Could you check a few things on this model? Use its own coordinates, in mm. Face numbers are marked on the shaded views. A direction names the side the tool comes from. Coordinates: 2 decimals unless noted, no trailing zeros. Order: outer loops, then holes, each group sorted by start corner. A loop starts at its lowest first (then second) coordinate and runs counter-clockwise, first axis right, second up. Notation, with made-up numbers: M 26,25.5 L 54,25.5 A32 ccw 54,52.5 Z; hole C -9,39 d3. An arc over 180 degrees is marked long. Write item = value, one per line. Start each with the question number.
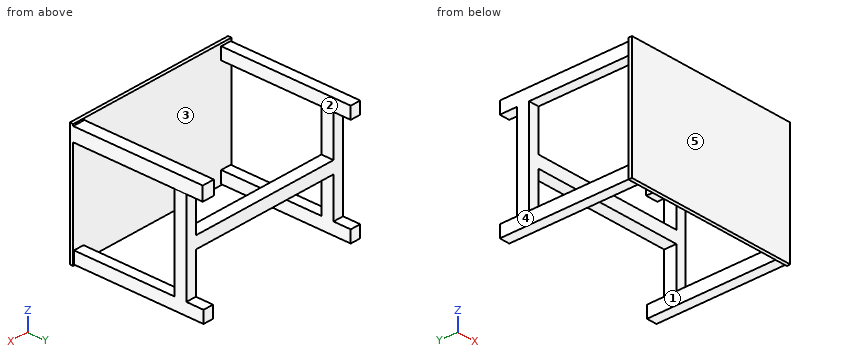
from build123d import *

# Parameters (mm, degrees)
SKETCH1_W           = 2000
SKETCH1_H           = 1400
BOSS_EXTRUDE1_DEPTH = 40
SKETCH4_W           = 120
SKETCH4_H           = 140
SKETCH4_W_2         = 140
SKETCH4_H_2         = 160
BOSS_EXTRUDE2_DEPTH = 1500
SKETCH5_W           = 120
SKETCH5_H           = 140
BOSS_EXTRUDE3_DEPTH = 1220
SKETCH6_W           = 140
SKETCH6_H           = 140
BOSS_EXTRUDE4_DEPTH = 1740


with BuildPart() as part:
    # Sketch1 → Boss-Extrude1 (new body)
    with BuildSketch(Plane(origin=(0, 0, 0), x_dir=(1, 0, 0), z_dir=(0, 1, 0))):
        Rectangle(SKETCH1_W, SKETCH1_H)
    extrude(amount=BOSS_EXTRUDE1_DEPTH)

    # Sketch4 → Boss-Extrude2 (add)
    with BuildSketch(Plane(origin=(0, 40, 0), x_dir=(1, 0, 0), z_dir=(0, 1, 0))):
        with Locations((-930, -600)):
            Rectangle(SKETCH4_W, SKETCH4_H)
        with Locations((930, 620)):
            Rectangle(SKETCH4_W, SKETCH4_H)
        with Locations((930, -600)):
            Rectangle(SKETCH4_W_2, SKETCH4_H_2)
        with Locations((-930, 620)):
            Rectangle(SKETCH4_W, SKETCH4_H)
    extrude(amount=BOSS_EXTRUDE2_DEPTH)

    # Sketch5 → Boss-Extrude3 (add)
    with BuildSketch(Plane.XY.offset(670)):
        with Locations((-930, 1270.83173518)):
            Rectangle(SKETCH5_W, SKETCH5_H)
        with Locations((930, 1270.83173518)):
            Rectangle(SKETCH5_W, SKETCH5_H)
    extrude(amount=-BOSS_EXTRUDE3_DEPTH)

    # Sketch6 → Boss-Extrude4 (add)
    with BuildSketch(Plane.ZY.offset(-870)):
        with Locations((-14.348286906, 1270.83173518)):
            Rectangle(SKETCH6_W, SKETCH6_H)
    extrude(amount=BOSS_EXTRUDE4_DEPTH)


solid = part.part
(1) Thinking about a two-plate mould opening in X: for the marked faces 3, 4 and 5, which applies, released by +X, released by -X, zero draft, split by the parting line, or undercut?
(2) Please list where these lines run through material, in increasing order: probe 1 along X at (y, z) = (1234, 143.5); probe 2 along Y at (x, z) = (-554.5, -581); probe 3 along Z at (x, y) = (897, 1283). Write a range as from..to.
(3) For the marked faces 1 and 2, which set-ups out of +Z, -Z, +X, -X, +Y, -Y let a thin tool reach every point of the face, with its end or its side?
(4) Imagine slicing it at C-C on z = 475. List the corners of the cut face in (x, y) for me, plus the area to 3 significant figures.
(5) Imagine slicing it at D-D on y = 1264.5. List the corners of the cut face in (x, z) for me, plus the area to 3 significant figures.
(6) Imagine slicing it at A-A on y = 921. List the corners of the cut face in (x, z) for me, plus the area to 3 significant figures.
(7) Will these pins go through, and if not, where does the flat tip stop? P1, Ø6, axis at x = 540, z = 460.5, coming from the +Y side; P2, Ø4, axis at x = 116.5, z = -49, coming from the +Y side.
(8) Imagine slicing it at B-B on x = -397.5. List the corners of the cut face in (y, z) for me.
Response:
q1.face_3 = undercut
q1.face_4 = released by -X
q1.face_5 = zero draft
q2.probe_1 = -990..-870, 870..990
q2.probe_2 = 0..40
q2.probe_3 = -690..680
q3.face_1 = -Z, +Y
q3.face_2 = +Z, +Y
q4.outline = M -1000,0 L 1000,0 L 1000,40 L -1000,40 Z; M -990,1200.83 L -870,1200.83 L -870,1340.83 L -990,1340.83 Z; M 870,1200.83 L 990,1200.83 L 990,1340.83 L 870,1340.83 Z
q4.area = 114,000 mm2
q5.outline = M -990,-690 L -870,-690 L -870,-84.35 L 870,-84.35 L 870,-690 L 990,-690 L 990,520 L 1000,520 L 1000,680 L 860,680 L 860,520 L 870,520 L 870,55.65 L -870,55.65 L -870,670 L -990,670 Z
q5.area = 574,000 mm2
q6.outline = M -990,-690 L -870,-690 L -870,-550 L -990,-550 Z; M -990,530 L -870,530 L -870,670 L -990,670 Z; M 860,520 L 1000,520 L 1000,680 L 860,680 Z; M 870,-690 L 990,-690 L 990,-550 L 870,-550 Z
q6.area = 72,800 mm2
q7.P1 = 40
q7.P2 = 1340.83
q8.outline = M 0,-700 L 40,-700 L 40,700 L 0,700 Z; M 1200.83,-84.35 L 1340.83,-84.35 L 1340.83,55.65 L 1200.83,55.65 Z
